```python
from build123d import *

# Parameters (mm, degrees)
BOSS_EXTRUDE1_DEPTH = 82.042
SKETCH2_R           = 3.175
CUT_EXTRUDE2_DEPTH  = 82.042
SKETCH3_R           = 3.175
CUT_EXTRUDE3_DEPTH  = 82.042


with BuildPart() as part:
    # Sketch1 → Boss-Extrude1 (new body)
    with BuildSketch(Plane.XY):
        Polygon((0, 0), (0, 25.4), (25.4, 25.4), (25.4, 22.225), (3.175, 22.225), (3.175, 0), align=None)
    extrude(amount=BOSS_EXTRUDE1_DEPTH)

    # Sketch2 → Cut-Extrude2 (cut)
    with BuildSketch(Plane.ZY):
        with Locations((70.9295, 12.7)):
            Circle(SKETCH2_R)
        with Locations((11.1125, 12.7)):
            Circle(SKETCH2_R)
    extrude(amount=-CUT_EXTRUDE2_DEPTH, mode=Mode.SUBTRACT)

    # Sketch3 → Cut-Extrude3 (cut)
    with BuildSketch(Plane(origin=(0, 25.4, 0), x_dir=(1, 0, 0), z_dir=(0, 1, 0))):
        with Locations(Location((12.7, -11.1125, 0), (0, 0, 270))):
            Circle(SKETCH3_R)
        with Locations(Location((12.7, -70.9295, 0), (0, 0, 270))):
            Circle(SKETCH3_R)
    extrude(amount=-CUT_EXTRUDE3_DEPTH, mode=Mode.SUBTRACT)


solid = part.part
```
Can you work these out from the model? Positions are in its coordinate system, mm. A direction names the side the tool comes from. Round coordinates to 2 decimals unless told otherwise and drop trailing zeros. Loops run counter-clockwise (first coordinate to the right, second up) from the corner with the lowest first, then second, coordinate; pieces in that order, holes last.
Item 1: Please list where these lines run through material, in increasing order: L1, parallel to Z at x = 11, y = 22.75; L2, parallel to X at y = 18.25, z = 45 (3 decimals); L3, parallel to Y at x = 6.5, z = 4 (3 decimals).
Item 2: Suppose I cut it at B-B, the plane x = 12.7. Write out the boundary of the cut face in (y, z) (1 decimal), then the cut area to 3 significant figures.
Item 3: Which directions (+Z, -Z, +X, -X, +Y, -Y) give clear straight access to the entire face, cutting with the end or side of a thin tool? Please do faces 1 (the flat face through (0, 13, 40)), 2 (the flat face through (3.175, 11, 40)).
Item 4: Will these pins go through, and if not, where does the flat tip stop? pin 1 Ø7.5 at (x, z) = (12.7, 11.11) entering from -Y (3 decimals); pin 2 Ø4 at (y, z) = (17, 18) entering from +X (3 decimals); pin 3 Ø5.5 at (x, z) = (12.7, 70.93) entering from -Y.
Item 5: Suppose I cut it at C-C, the plane z = 71.5. Write out the boundary of the cut face in (x, y) (3 decimals).
Item 6: Suppose I cut it at D-D, the plane y = 4. Write out the boundary of the cut face in (x, z) (3 decimals).
Item 7: Suppose I cut it at A-A, the plane y = 12.7. Write out the boundary of the cut face in (x, z) (1 decimal).
Item 8: If we mould it in two halves opening along Y, with no side actions, what happens to faces 3 (the flat face through (14, 22.225, 40)), 4 (the flat face through (8, 23, 82.042)), 5 (the cylindrical face through (1.57, 13.65, 73.96))? For each: +Y half, -Y half, draft (parallel to the pull), parting line (faces both ways), or undercut.
Reported:
1. L1: z = 0 to 8.43, 13.79 to 68.25, 73.61 to 82.04
1. L2: x = 0 to 3.175
1. L3: y = 22.225 to 25.4
2. outline: (22.2, 0) - (25.4, 0) - (25.4, 7.9) - (22.2, 7.9) - close; (22.2, 14.3) - (25.4, 14.3) - (25.4, 67.8) - (22.2, 67.8) - close; (22.2, 74.1) - (25.4, 74.1) - (25.4, 82) - (22.2, 82) - close
2. area: 220 mm2
3. face 1: +Z, -Z, -X, +Y, -Y
3. face 2: +Z, -Z, +X, -Y
4. pin 1: stops at y = 22.225
4. pin 2: stops at x = 3.175
4. pin 3: passes through
5. outline: (0, 0) - (3.175, 0) - (3.175, 9.577) - (0, 9.577) - close; (0, 15.823) - (3.175, 15.823) - (3.175, 22.225) - (9.577, 22.225) - (9.577, 25.4) - (0, 25.4) - close; (15.823, 22.225) - (25.4, 22.225) - (25.4, 25.4) - (15.823, 25.4) - close
6. outline: (0, 0) - (3.175, 0) - (3.175, 82.042) - (0, 82.042) - close
7. outline: (0, 0) - (3.2, 0) - (3.2, 7.9) - (0, 7.9) - close; (0, 14.3) - (3.2, 14.3) - (3.2, 67.8) - (0, 67.8) - close; (0, 74.1) - (3.2, 74.1) - (3.2, 82) - (0, 82) - close
8. face 3: -Y half
8. face 4: draft
8. face 5: undercut
